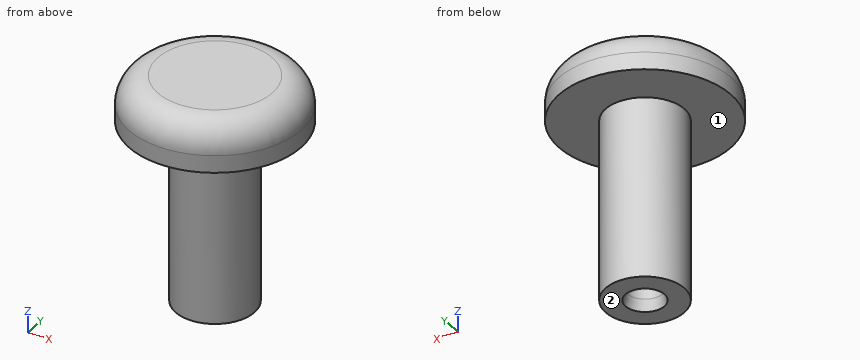
```python
from build123d import *

# Parameters (mm, degrees)
SKETCH1_R           = 3.4375
BOSS_EXTRUDE1_DEPTH = 15.7
SKETCH2_R           = 7.5
BOSS_EXTRUDE2_DEPTH = 4
SKETCH3_R           = 1.5
CUT_EXTRUDE1_DEPTH  = 5
CHAMFER1_SIZE       = 0.2
CHAMFER1_SIZE2      = 1
FILLET1_R           = 2.5


with BuildPart() as part:
    # Sketch1 → Boss-Extrude1 (new body)
    with BuildSketch(Plane.XY):
        Circle(SKETCH1_R)
    extrude(amount=BOSS_EXTRUDE1_DEPTH)

    # Sketch2 → Boss-Extrude2 (add)
    with BuildSketch(Plane.XY.offset(15.7)):
        Circle(SKETCH2_R)
    extrude(amount=BOSS_EXTRUDE2_DEPTH)

    # Sketch3 → Cut-Extrude1 (cut)
    with BuildSketch(Plane(origin=(0, 0, 0), x_dir=(-1, 0, 0), z_dir=(0, 0, -1))):
        Circle(SKETCH3_R)
    extrude(amount=-CUT_EXTRUDE1_DEPTH, mode=Mode.SUBTRACT)

    # Chamfer1
    chamfer1_edges = [part.edges().sort_by_distance(p)[0] for p in [
        (1.5, 0, 0),
    ]]
    chamfer1_side = [part.faces().sort_by_distance(p)[0] for p in [
        (-3.340272818, 0, 0),
    ]]
    chamfer(chamfer1_edges, length=CHAMFER1_SIZE, length2=CHAMFER1_SIZE2, reference=chamfer1_side[0])

    # Fillet1
    fillet1_edges = [part.edges().sort_by_distance(p)[0] for p in [
        (-7.5, 0, 19.7),
    ]]
    fillet(fillet1_edges, radius=FILLET1_R)


solid = part.part
```
Could you check a few things on this model? Use its own coordinates, in mm. Face numbers are marked on the shaded views. A direction names the side the tool comes from. Coordinates: 2 decimals unless noted, no trailing zeros. Write each loop counter-clockwise with the first axis right and the second up, starting at its lowest first coordinate (ties: lowest second). Pieces come first, ordered by that corner, then holes. Notation, with made-up numbers: (21.25, -12) -> (42.25, -12) arc R31 ccw to (42.25, 20) -> close; hole circle Ø7 at (-7, 12.25). An arc over 180 degrees is marked (long way). One line per question, with ' | ' between items. Start each with the question number.
1. If we section it at D-D (z = 15): Please give me the cut outline in (x, y) (1 decimal).
2. For the marked faces 1 and 2, which set-ups out of +Z, -Z, +X, -X, +Y, -Y let a thin tool reach every point of the face, with its end or its side?
3. Please list where these lines run through material, in increasing order: line 1 along Y through (x, z) = (0, 2.75); line 2 along Z through (x, y) = (1.75, 4.25); line 3 along Z through (x, y) = (-5.5, -2).
4. If we section it at A-A (z = 4.75): Please give me the cut outline in (x, y) (1 decimal), and give its area (3 significant figures).
5. Will these pins go through, and if not, where does the flat tip stop? P1, Ø4, axis at x = -3, y = -5, coming from the -Z side; P2, Ø1, axis at x = 0.5, z = 6.5, coming from the +Y side; P3, Ø8, axis at x = 5.5, z = 9, coming from the +Y side.
6. If we section it at B-B (y = 0): Please give me the cut outline in (x, z), and give its area (3 significant figures).
Return value:
1) outline: circle Ø6.9 at (0, 0)
2) face 1: -Z | face 2: -Z, +X, -X, +Y, -Y
3) line 1: y = -3.44 to -1.5, 1.5 to 3.44 | line 2: z = 15.7 to 19.7 | line 3: z = 15.7 to 19.55
4) outline: circle Ø6.9 at (0, 0); hole circle Ø3 at (0, 0) | area: 30.1 mm²
5) P1: stops at z = 15.7 | P2: stops at y = 3.44 | P3: stops at y = 3.09
6) outline: (-7.5, 15.7) -> (-3.44, 15.7) -> (-3.44, 0) -> (-1.7, 0) -> (-1.5, 1) -> (-1.5, 5) -> (1.5, 5) -> (1.5, 1) -> (1.7, 0) -> (3.44, 0) -> (3.44, 15.7) -> (7.5, 15.7) -> (7.5, 17.2) arc R2.5 ccw to (5, 19.7) -> (-5, 19.7) arc R2.5 ccw to (-7.5, 17.2) -> close | area: 150 mm²
